Verification items for the finished model (mm, model axes). Give positions to 0.01 mm unless a question says otherwise; leave off trailing zeros. Write each loop counter-clockwise with the first axis right and the second up, starting at its lowest first coordinate (ties: lowest second). Pieces come first, ordered by that corner, then holes. Notation, with made-up numbers: (27, 55.25) - (38, 55.25) arc R17 ccw to (38, 76.25) - close; hole circle Ø3 at (-12.5, 77). An arc over 180 degrees is marked (long way). Put each result on its own line as item: value.
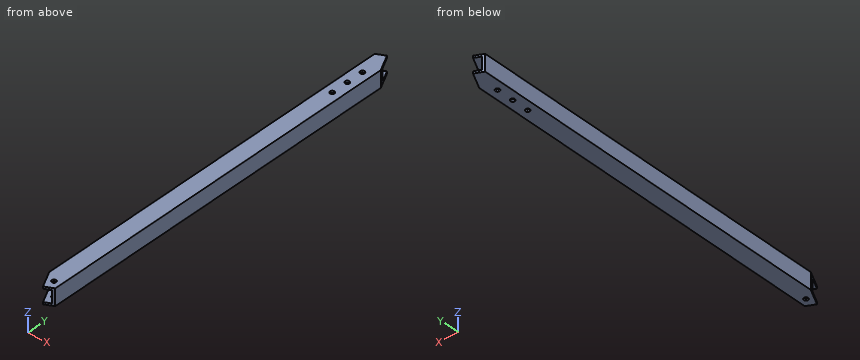
Autodesk Inventor part; units mm, degrees
ref_plane "YZ Plane" through (0, 0, 0) normal (1, 0, 0) x (0, 1, 0)
ref_plane "XZ Plane" through (0, 0, 0) normal (0, 1, 0) x (-1, 0, 0)
ref_plane "XY Plane" through (0, 0, 0) normal (0, 0, 1) x (1, 0, 0)
sketch "Sketch1" plane through (0, 0, 0) normal (0, 1, 0) x (-1, 0, 0)
  line L0 (-12.7, -12.7) -> (12.7, -12.7)
  line L1 (12.7, -12.7) -> (12.7, 12.7)
  line L2 (12.7, 12.7) -> (-12.7, 12.7)
  line L3 (-12.7, 12.7) -> (-12.7, -12.7)
  line L4 (-12.7, -12.7) -> (12.7, 12.7) construction
  line L5 (12.7, -12.7) -> (-12.7, 12.7) construction
  line L6 (9.525, 9.525) -> (9.525, -9.525)
  line L7 (9.525, -9.525) -> (-9.525, -9.525)
  line L8 (-9.525, -9.525) -> (-9.525, 9.525)
  line L9 (-9.525, 9.525) -> (9.525, 9.525)
  point P0 (0, 0)
  dimension "d0" = 25.4
  dimension "d1" = 25.4
  dimension "d2" = 3.175
extrude "Extrusion1" add sketch "Sketch1" along normal blind 579.374
sketch "Sketch4" plane through (-12.7, 0, 12.7) normal (0, 0, 1) x (1, 0, 0)
  line L0 (249.4631, 122.7685) -> (12.7, 579.374)
  line L1 (12.7, 579.374) -> (-224.0631, 456.6055)
  line L2 (-224.0631, 456.6055) -> (12.7, 0)
  line L3 (12.7, 0) -> (249.4631, 122.7685)
  line L4 (0, 0) -> (25.4, 0)
  line L5 (0, 579.374) -> (25.4, 579.374)
  line L6 (0, 0) -> (25.4, 0)
  line L7 (25.4, 0) -> (25.4, 579.374)
  line L8 (0, 579.374) -> (25.4, 579.374)
  line L9 (0, 0) -> (0, 579.374)
  point P0 (0, 24.4924)
  point P1 (25.4, 6.5853)
  point P2 (0, 572.7887)
  point P3 (25.4, 554.8816)
  dimension "d13" = 266.7
extrude "Extrusion4" cut sketch "Sketch4" against normal blind 370.4968 contours L0 L5 L7 | L7 L4 L3 | L1 L9 L5 | L4 L9 L2
sketch "Sketch6" plane through (12.7, 6.5853, 12.7) normal (0, 0, 1) x (1, 0, 0)
  line L0 (-24.3922, 15.9636) -> (-46.9411, 4.2713) construction
  line L1 (-46.9411, 4.2713) -> (-35.2489, -18.2776) construction
  line L2 (-35.2489, -18.2776) -> (-12.7, -6.5853) construction
  line L3 (-12.7, -6.5853) -> (-25.4, 17.9071) construction
  line L4 (-25.4, 17.9071) -> (-12.7, -6.5853) construction
  line L5 (-46.9411, 4.2713) -> (-12.7, -6.5853) construction
  circle A0 centre (-29.8206, -1.157) radius 3.2512 construction
  circle A1 centre (-10.0903, 9.0737) radius 3.2512
  line L6 (-41.095, -7.0031) -> (-4.5992, 11.921) construction
  dimension "d21" = 25.4
  dimension "d22" = 25.4
  dimension "d23" = 6.5024
  dimension "d24" = 6.5024
  dimension "d25" = 22.225
extrude "Extrusion6" cut sketch "Sketch6" against normal blind 25.4
sketch "Sketch7" plane through (12.7, 6.5853, 12.7) normal (0, 0, 1) x (1, 0, 0)
  line L0 (0, 548.2963) -> (-12.7, 572.7887) construction
  line L1 (-12.7, 572.7887) -> (36.992, 476.956) construction
  line L2 (36.992, 476.956) -> (59.5409, 488.6482) construction
  line L3 (59.5409, 488.6482) -> (9.8489, 584.4809) construction
  line L4 (9.8489, 584.4809) -> (-12.7, 572.7887) construction
  circle A0 centre (42.4203, 494.0765) radius 3.2512 construction
  circle A1 centre (30.7281, 516.6254) radius 3.2512 construction
  circle A2 centre (19.0359, 539.1743) radius 3.2512 construction
  line L5 (48.2665, 482.8021) -> (-1.4256, 578.6348) construction
  line L6 (0, 0) -> (0, 548.2963) construction
  line L7 (0, 548.2963) -> (-6.7276, 575.8856) construction
  circle A3 centre (-12.7, 480.6356) radius 3.2512
  circle A4 centre (-12.7, 506.0356) radius 3.2512
  circle A5 centre (-12.7, 531.4356) radius 3.2512
  point P0 (-12.7, -6.5853)
  dimension "d28" = 25.4
  dimension "d29" = 107.95
  dimension "d30" = 6.5024
  dimension "d31" = 44.45
  dimension "d32" = 25.4
  dimension "d33" = 25.4
  dimension "d34" = 27.408
  dimension "d35" = 166.296
extrude "Extrusion7" cut sketch "Sketch7" against normal blind 25.4
properties part number "STRU_013_BilletCrossbar2_Angled" material "Aluminum 6061"
Q1. Section check B-B, the plane z = -1.75. Record the cut outline in (x, y) (3 decimals).
Answers follow:
outline: (-12.7, 24.492) - (-9.525, 18.369) - (-9.525, 574.435) - (-12.7, 572.789) - close; (9.525, 4.939) - (12.7, 6.585) - (12.7, 554.882) - (9.525, 561.005) - close
Q2. Section check A-A, the plane y = 284. Record the cut outline in (x, z) (3 decimals).
Answers follow:
outline: (-12.7, -12.7) - (12.7, -12.7) - (12.7, 12.7) - (-12.7, 12.7) - close; hole (-9.525, -9.525) - (9.525, -9.525) - (9.525, 9.525) - (-9.525, 9.525) - close
Q3. Scan lines: line 1 along X through (y, z) = (124.5, 6) (3 decimals); line 2 along Y through (x, z) = (3, 9.75). Record each from-to range of solid material in increasing order.
Answers follow:
line 1: x = -12.7 to -9.525, 9.525 to 12.7
line 2: y = 1.56 to 12.43, 18.89 to 485.97, 488.47 to 511.37, 513.87 to 536.77, 539.27 to 573.59
Q4. Go/stop test with a flat-tipped pin: pin 1 Ø1 at (x, z) = (-10, -6) entering from +Y (3 decimals). Record where the tip stops, or that it passes through.
Answers follow:
pin 1: stops at y = 574.435
